```python
from build123d import *

# Parameters (mm, degrees)
F0_W     = 60
F0_H     = 60
F1_DEPTH = 10
F3_D     = 5.5


with BuildPart() as f1:
    # F0 (on Top) → F1 (new body)
    with BuildSketch(Plane.XY):
        Rectangle(F0_W, F0_H)
    extrude(amount=-F1_DEPTH)

    # F3 (through all)
    with Locations(Plane.XY):
        with Locations((23, -22.3507442691), (-23, -22.3507442691), (-23, 23.6492557309), (23, 23.6492557309)):
            Hole(F3_D / 2)


solid = f1.part
```
Source: CAD feature listing. Evaluate the final solid. Frame: model axes, mm. Round coordinates to 2 decimals unless told otherwise and drop trailing zeros. Write each loop counter-clockwise with the first axis right and the second up, starting at its lowest first coordinate (ties: lowest second). Pieces come first, ordered by that corner, then holes. Notation, with made-up numbers: M 65,27.5 L 101,27.5 A18 ccw 101,32.5 Z; hole C -39,32 d4. An arc over 180 degrees is marked long. Use CSV: the item, a comma, the result in double quotes. Start each with the question number.
Q1. Pull-direction query (Y, two-part tool) for faces 1 (the face through (0, -30, -5)), 2 (the face through (30, 0, -5)), 3 (the face through (-20.253, 23.77, -5.07)); classes: +Y half, -Y half, draft (parallel to the pull), parting line (faces both ways), or undercut.
Q2. Cut plane A-A on x = 23. Output: boundary loops of the cut face in (y, z), plus the area to 3 significant figures.
Q3. Cut plane B-B on y = 24.5. Output: boundary loops of the cut face in (x, z), plus the area to 3 significant figures.
Q4. Cut plane C-C on z = -3.5. Output: boundary loops of the cut face in (x, y), plus the area to 3 significant figures.
Q5. Line query: line 1 (Y direction, x = 23, z = -3); line 2 (Y direction, x = 21, z = -3). Output: solid intervals per line, ascending. Write a range as from..to.
Results found:
1,face 1,"-Y half"
1,face 2,"draft"
1,face 3,"undercut"
2,outline,"M -30,-10 L -25.1,-10 L -25.1,0 L -30,0 Z; M -19.6,-10 L 20.9,-10 L 20.9,0 L -19.6,0 Z; M 26.4,-10 L 30,-10 L 30,0 L 26.4,0 Z"
2,area,"490 mm^2"
3,outline,"M -30,-10 L -25.62,-10 L -25.62,0 L -30,0 Z; M -20.38,-10 L 20.38,-10 L 20.38,0 L -20.38,0 Z; M 25.62,-10 L 30,-10 L 30,0 L 25.62,0 Z"
3,area,"495 mm^2"
4,outline,"M -30,-30 L 30,-30 L 30,30 L -30,30 Z; hole C -23,-22.35 d5.5; hole C -23,23.65 d5.5; hole C 23,-22.35 d5.5; hole C 23,23.65 d5.5"
4,area,"3,500 mm^2"
5,line 1,"-30..-25.1, -19.6..20.9, 26.4..30"
5,line 2,"-30..-24.24, -20.46..21.76, 25.54..30"
